Read the model definition and answer for the solid it produces. Units are mm, in the model's axes. A direction names the side the tool comes from. Coordinates: 2 decimals unless noted, no trailing zeros. Write each loop counter-clockwise with the first axis right and the second up, starting at its lowest first coordinate (ties: lowest second). Pieces come first, ordered by that corner, then holes. Notation, with made-up numbers: M 30.25,24 L 77.25,24 A23 cw 77.25,60 Z; hole C 51,16.5 d1. An arc over 180 degrees is marked long. Write item = value, one per line.
from build123d import *


with BuildPart() as part:
    # Sketch1 → Revolve1 (revolve)
    with BuildSketch(Plane(origin=(0, 0, 0), x_dir=(0, 0, -1), z_dir=(1, 0, 0))):
        with BuildLine():
            Line((-13.1, 6), (-12.5, 5.4))
            Line((-12.5, 5.4), (-12.5, -5.4))
            Line((-12.5, -5.4), (-13.1, -6))
            Line((-13.1, -6), (-16, -6))
            Line((-16, -6), (-16, -5.25))
            Line((-16, -5.25), (-21.25, -5.25))
            Line((-21.25, -5.25), (-21.25, -6))
            Line((-21.25, -6), (-22.9, -6))
            ThreePointArc((-22.9, -6), (-23.324264069, -5.824264069), (-23.5, -5.4))
            Line((-23.5, -5.4), (-23.5, 5.4))
            ThreePointArc((-23.5, 5.4), (-23.324264069, 5.824264069), (-22.9, 6))
            Line((-22.9, 6), (-21.25, 6))
            Line((-21.25, 6), (-21.25, 5.25))
            Line((-21.25, 5.25), (-16, 5.25))
            Line((-16, 5.25), (-16, 6))
            Line((-16, 6), (-13.1, 6))
        make_face()
    revolve(axis=Axis((0, 26.680665717, 0), (0, -1, 0)))


solid = part.part
Item 1: Flat-ended cylindrical pins translate along their axes: pin 1 (1 mm diameter, centred on x = 15.5, y = -3.5, fed in from -Z); pin 2 (15 mm diameter, centred on x = 0, z = 0, fed in from -Y); pin 3 (1.5 mm diameter, centred on x = 16.5, z = -4.5, fed in from -Y); pin 4 (2 mm diameter, centred on y = -4.5, z = 6, fed in from +X). Find the tip coordinate at first contact, or state that the pin passes through.
Worked answers:
pin_1 = -18.09
pin_2 = through
pin_3 = -5.25
pin_4 = 22.96
Item 2: Consider line 1 along X through (y, z) = (-2, 0); line 2 along X through (y, z) = (5.8, 0). Determine where each line is inside the solid, lowest interval first. Write a range as from..to.
Worked answers:
line_1 = -23.5..-12.5, 12.5..23.5
line_2 = -23.35..-21.25, -16..-12.9, 12.9..16, 21.25..23.35
Item 3: Find section C-C (y = -1). Determine the outline of the cut face in (x, z), and give its area (3 significant figures).
Worked answers:
outline = C 0,0 d47; hole C 0,0 d25
area = 1,240 mm²
Item 4: For a pull along Z with two mould halves and no side action, classify faces 1 (the face through (-7.1, 0.1, 22.4)), 2 (the face through (12, -6, 6)), 3 (the face through (15.62, -5.62, -3.47)) as released by +Z, released by -Z, zero draft, split by the parting line, or undercut.
Worked answers:
face_1 = split by the parting line
face_2 = zero draft
face_3 = undercut
Item 5: Which of the six approach directions +Z, -Z, +X, -X, +Y, -Y give full straight-line access (tool end or side, diameter ignored) to faces 4 (the face through (15.2, 6, 15.2)), 5 (the face through (-16, -5.25, -3)), 6 (the face through (15.62, 5.63, -3.47))?
Worked answers:
face_4 = +Z, -Z, +X, -X, +Y
face_5 = -Y
face_6 = +Y
